from build123d import *

# Parameters (mm, degrees)
SKETCH1_R               = 53.721
SKETCH1_R_2             = 50.8
EXTRUDE_THIN1_DEPTH     = 50.8
CUT_EXTRUDE1_REACH      = 132.424
CUT_EXTRUDE1_END_RADIUS = 50.8
SKETCH2_R               = 1.6383
CIRPATTERN1_COUNT       = 8


with BuildPart() as part:
    # Sketch1 → Extrude-Thin1 (new body)
    with BuildSketch(Plane(origin=(0, 0, 0), x_dir=(1, 0, 0), z_dir=(0, 1, 0))):
        Circle(SKETCH1_R)
        Circle(SKETCH1_R_2, mode=Mode.SUBTRACT)
    extrude(amount=EXTRUDE_THIN1_DEPTH)

    # Cut-Extrude1: up to this cylinder (the profile starts outside it)
    cut_extrude1_end = Plane(origin=(0, 25.4, 0), z_dir=(0, -1, 0)) * Cylinder(CUT_EXTRUDE1_END_RADIUS, 367.448, mode=Mode.PRIVATE)
    # Sketch2 → Cut-Extrude1 (cut, up to the surface)
    with BuildSketch(Plane.XY.offset(53.721), mode=Mode.PRIVATE) as cut_extrude1_sk1:
        with Locations((0, 25.4)):
            Circle(SKETCH2_R)
    cut_extrude1_tool1 = extrude(cut_extrude1_sk1.sketch, amount=-CUT_EXTRUDE1_REACH, mode=Mode.PRIVATE) - cut_extrude1_end
    cut_extrude1 = cut_extrude1_tool1.solids().sort_by_distance((0, 25.4, 53.721))[0]
    add(cut_extrude1, mode=Mode.SUBTRACT)

    # CirPattern1: Cut-Extrude1 ×8 about axis
    cirpattern1_axis = Axis((0, 50.8, 0), (0, -1, 0))
    for i in range(1, CIRPATTERN1_COUNT):
        add(cut_extrude1.rotate(cirpattern1_axis, i * 360 / CIRPATTERN1_COUNT), mode=Mode.SUBTRACT)


solid = part.part
Here's how the part is built. I have some questions about the finished solid (model axes, mm). Round coordinates to 2 decimals unless told otherwise and drop trailing zeros. Order: outer loops, then holes, each group sorted by start corner. A loop starts at its lowest first (then second) coordinate and runs counter-clockwise, first axis right, second up. Notation, with made-up numbers: M -14.5,62 L -2.5,62 A17 cw -2.5,71 Z; hole C -29.5,70 d4. An arc over 180 degrees is marked long. One line per question, with ' | ' between items.
1) Imagine slicing it at A-A, the plane x = 0. Write out the boundary of the cut face in (y, z).
Checked values:
outline: M 0,-53.72 L 23.76,-53.72 L 23.76,-50.8 L 0,-50.8 Z; M 0,50.8 L 23.76,50.8 L 23.76,53.72 L 0,53.72 Z; M 27.04,-53.72 L 50.8,-53.72 L 50.8,-50.8 L 27.04,-50.8 Z; M 27.04,50.8 L 50.8,50.8 L 50.8,53.72 L 27.04,53.72 Z
2) I'm going to push flat-ended pins straight in: pin 1 Ø4 at (y, z) = (17, 42.5) entering from -X; pin 2 Ø2 at (y, z) = (25.4, 0) entering from -X; pin 3 Ø1.5 at (x, y) = (-21, 38.5) entering from -Z; pin 4 Ø10 at (x, y) = (9, 8.5) entering from -Z. Where does each tip first touch, or does it pass through?
Checked values:
pin 1: stops at x = -35.29 | pin 2: passes through | pin 3: stops at z = -49.76 | pin 4: stops at z = -53.57
3) Imagine slicing it at D-D, the plane z = 25. Write out the boundary of the cut face in (x, y).
Checked values:
outline: M -47.55,0 L -44.22,0 L -44.22,50.8 L -47.55,50.8 Z; M 44.22,0 L 47.55,0 L 47.55,50.8 L 44.22,50.8 Z
4) We'd pull the mould along Z, two halves only. Please class faces 1 (the cylindrical face through (46.926, 25.044, 19.457)), 2 (the flat face through (40, 50.8, -32)), 3 (the cylindrical face through (-6.993, 25.044, -53.264)), 4 (the cylindrical face through (-36.105, 26.507, -37.813)): released by +Z, released by -Z, zero draft, split by the parting line, or undercut.
Checked values:
face 1: undercut | face 2: zero draft | face 3: split by the parting line | face 4: undercut
5) I need wall thicknesses on line 1 (Y direction, x = 0, z = -52.95); line 2 (X direction, y = 40, z = 0); line 3 (Z direction, x = -21, y = 9). Which ranges of each line are inside material? Lowest first, please.
Checked values:
line 1: y = 0 to 23.76, 27.04 to 50.8 | line 2: x = -53.72 to -50.8, 50.8 to 53.72 | line 3: z = -49.45 to -46.26, 46.26 to 49.45
6) Imagine slicing it at C-C, the plane x = 31.5. Write out the boundary of the cut face in (y, z), plus the area to 3 significant figures.
Checked values:
outline: M 0,-43.52 L 50.8,-43.52 L 50.8,-39.85 L 0,-39.85 Z; M 0,39.85 L 50.8,39.85 L 50.8,43.52 L 0,43.52 Z | area: 372 mm²
7) Imagine slicing it at B-B, the plane z = 0. Write out the boundary of the cut face in (x, y).
Checked values:
outline: M -53.72,0 L -50.8,0 L -50.8,23.76 L -53.72,23.76 Z; M -53.72,27.04 L -50.8,27.04 L -50.8,50.8 L -53.72,50.8 Z; M 50.8,0 L 53.72,0 L 53.72,23.76 L 50.8,23.76 Z; M 50.8,27.04 L 53.72,27.04 L 53.72,50.8 L 50.8,50.8 Z
